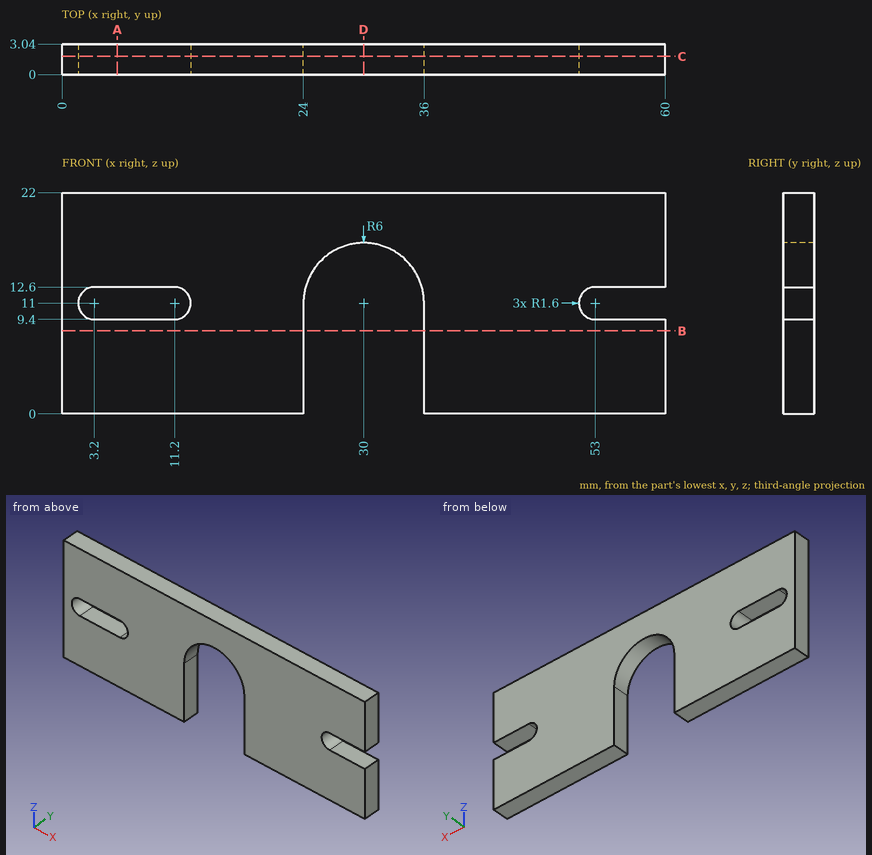
Design review of the part shown in the three views and the two pictorial views. Dimensions are in mm from the part's minimum x, y and z. Give positions to 0.01 mm unless a question says otherwise; leave off trailing zeros. Loops run counter-clockwise (first coordinate to the right, second up) from the corner with the lowest first, then second, coordinate; pieces in that order, holes last. Notation, with made-up numbers: (-30.75, 25.5) - (-10.75, 25.5) arc R17 ccw to (-10.75, 39.5) - close; hole circle Ø11 at (-17, 44). An arc over 180 degrees is marked (long way). Answer as a JSON object with one key per item and string values.
Q1. Add section A-A on x = 5.5. State the section outline as (y, z) points.
Worked out:
{"outline": "(0, 0) - (3.04, 0) - (3.04, 9.4) - (0, 9.4) - close; (0, 12.6) - (3.04, 12.6) - (3.04, 22) - (0, 22) - close"}
Q2. Add section B-B on z = 8.25. State the section outline as (x, y) points.
Worked out:
{"outline": "(0, 0) - (24, 0) - (24, 3.04) - (0, 3.04) - close; (36, 0) - (60, 0) - (60, 3.04) - (36, 3.04) - close"}
Q3. Insertion check: pin 1 (0.9 mm diameter, centred on x = 7.5, y = 1, fed in from -Z). The pin has a flat end and moves straight along its axis. Give the tip position at first contact, or say it passes through.
Worked out:
{"pin 1": "stops at z = 0"}
Q4. To check wall thickness, follow line 1 along X through (y, z) = (2.6, 1.75); line 2 along Z through (x, y) = (7.5, 0.5); line 3 along X through (y, z) = (2.35, 13). State the ranges of each line that lie inside material, in increasing order.
Worked out:
{"line 1": "x = 0 to 24, 36 to 60", "line 2": "z = 0 to 9.4, 12.6 to 22", "line 3": "x = 0 to 24.34, 35.66 to 60"}
Q5. Add section C-C on y = 1.8. State the section outline as (x, z) points.
Worked out:
{"outline": "(0, 0) - (24, 0) - (24, 11) arc R6 cw to (36, 11) - (36, 0) - (60, 0) - (60, 9.4) - (53, 9.4) arc R1.6 cw to (53, 12.6) - (60, 12.6) - (60, 22) - (0, 22) - close; hole (3.2, 9.4) - (11.2, 9.4) arc R1.6 ccw to (11.2, 12.6) - (3.2, 12.6) arc R1.6 ccw to start"}
Q6. Add section D-D on x = 30. State the section outline as (y, z) points.
Worked out:
{"outline": "(0, 17) - (3.04, 17) - (3.04, 22) - (0, 22) - close"}
